Geometry: final body of the model. Coordinates: model frame, mm. Round coordinates to 2 decimals unless told otherwise and drop trailing zeros. Loops run counter-clockwise (first coordinate to the right, second up) from the corner with the lowest first, then second, coordinate; pieces in that order, holes last. Notation, with made-up numbers: M 71.25,58.5 L 107.25,58.5 A28 cw 107.25,81.5 Z; hole C 38,-27 d10. An arc over 180 degrees is marked long. Answer as a JSON object with one key per item and string values.
```python
from build123d import *

# Parameters (mm, degrees)
PAD003_DEPTH    = 9.525
SKETCH090_R     = 2.8575
POCKET018_DEPTH = 6.096
SKETCH091_R     = 2.8575
POCKET019_DEPTH = 6.096
SKETCH092_R     = 2.8575
POCKET020_DEPTH = 6.096
SKETCH093_R     = 2.8575
POCKET021_DEPTH = 6.096
SKETCH111_R     = 1.778
POCKET035_DEPTH = 9.526
SKETCH112_R     = 2.794
POCKET036_DEPTH = 3.048


with BuildPart() as part:
    # Sketch005 → Pad003 (new body)
    with BuildSketch(Plane.XZ):
        Polygon((66.675, -19.05), (66.675, 19.05), (-53.975, 19.05), (-53.975, 6.35), (-66.675, 6.35), (-66.675, -6.35), (-53.975, -6.35), (-53.975, -19.05), align=None)
    extrude(amount=PAD003_DEPTH)

    # Sketch090 (on Face6 of Pad003) → Pocket018 (cut)
    with BuildSketch(Plane(origin=(0, 0, 19.05), x_dir=(-1, 0, 0), z_dir=(0, 0, 1))):
        with Locations((38.1, 4.7625)):
            Circle(SKETCH090_R)
        with Locations((-38.1, 4.7625)):
            Circle(SKETCH090_R)
    extrude(amount=-POCKET018_DEPTH, mode=Mode.SUBTRACT)

    # Sketch091 (on Face4 of Pad003) → Pocket019 (cut)
    with BuildSketch(Plane(origin=(0, 0, -19.05), x_dir=(1, 0, 0), z_dir=(0, 0, -1))):
        with Locations((38.1, 4.7625)):
            Circle(SKETCH091_R)
        with Locations((-38.1, 4.7625)):
            Circle(SKETCH091_R)
    extrude(amount=-POCKET019_DEPTH, mode=Mode.SUBTRACT)

    # Sketch092 (on Face9 of Pocket019) → Pocket020 (cut)
    with BuildSketch(Plane(origin=(66.675, 0, 0), x_dir=(0, 0, 1), z_dir=(1, 0, 0))):
        with Locations((12.7, 4.7625)):
            Circle(SKETCH092_R)
        with Locations((-12.7, 4.7625)):
            Circle(SKETCH092_R)
    extrude(amount=-POCKET020_DEPTH, mode=Mode.SUBTRACT)

    # Sketch093 (on Face1 of Pocket019) → Pocket021 (cut)
    with BuildSketch(Plane(origin=(-66.675, 0, 0), x_dir=(0, 0, -1), z_dir=(-1, 0, 0))):
        with Locations((0, 4.7625)):
            Circle(SKETCH093_R)
    extrude(amount=-POCKET021_DEPTH, mode=Mode.SUBTRACT)

    # Sketch111 (on Face4 of Pocket021) → Pocket035 (cut, through all)
    with BuildSketch(Plane.XZ.offset(9.525)):
        with Locations((-20.828, 7.9375)):
            Circle(SKETCH111_R)
        with Locations((-20.828, -7.9375)):
            Circle(SKETCH111_R)
    extrude(amount=-POCKET035_DEPTH, mode=Mode.SUBTRACT)

    # Sketch112 (on Face4 of Pocket035) → Pocket036 (cut)
    with BuildSketch(Plane.XZ.offset(9.525)):
        with Locations((-20.828, 7.9375)):
            Circle(SKETCH112_R)
        with Locations((-20.828, -7.9375)):
            Circle(SKETCH112_R)
    extrude(amount=-POCKET036_DEPTH, mode=Mode.SUBTRACT)


with BuildPart() as part_1:
    # Body003 placement: moved
    add(part.part.moved(Location((-66.7258, -20.066, 0))))


solid = part_1.part
```
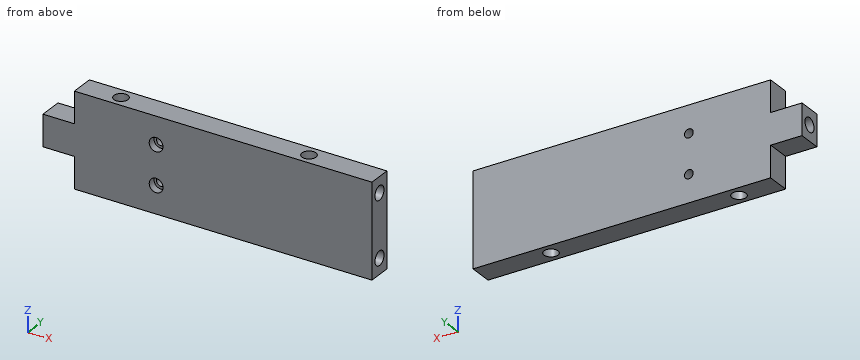
1) Line query: probe 1 along X at (y, z) = (-23.75, 8.5); probe 2 along X at (y, z) = (-27, 9); probe 3 along X at (y, z) = (-29, -16.5). Output: solid intervals per line, ascending.
Geometry results:
{"probe 1": "-120.7 to -89.24, -85.87 to -0.05", "probe 2": "-120.7 to -90.14, -84.97 to -0.05", "probe 3": "-120.7 to -0.05"}
2) First-contact query: pin 1 (5 mm diameter, centred on y = -23.5, z = 16, fed in from -X); pin 2 (3.5 mm diameter, centred on y = -24.83, z = 12.7, fed in from +X); pin 3 (3 mm diameter, centred on x = -129.5, y = -23.5, fed in from -Z). Flat tips, straight axial feed; report the tip coordinate or a pass-through.
Geometry results:
{"pin 1": "x = -120.7", "pin 2": "x = -6.15", "pin 3": "z = -6.35"}
3) Cut plane B-B on y = -23.5. Count the separate pieces of the cut face and the enclosed holes in it, and give its area (3 significant figures).
Geometry results:
{"separate pieces": "1", "enclosed holes": "2", "area": "4,520 mm2"}
4) Cut plane A-A on z = 0. Return the cut outline in (x, y).
Geometry results:
{"outline": "M -133.4,-29.59 L -0.05,-29.59 L -0.05,-20.07 L -133.4,-20.07 L -133.4,-21.97 L -127.3,-21.97 L -127.3,-27.69 L -133.4,-27.69 Z"}
